Can you work these out from the model? Positions are in its coordinate system, mm. Face numbers are marked on the shaded views. Coordinates: 2 decimals unless noted, no trailing zeros. Order: outer loops, then holes, each group sorted by start corner. A loop starts at its lowest first (then second) coordinate and runs counter-clockwise, first axis right, second up. Notation, with made-up numbers: (74.25, 72) - (111.25, 72) arc R15 ccw to (111.25, 93) - close; hole circle Ø8 at (-5.5, 28.25). An arc over 180 degrees is marked (long way). Return JSON: item names as keys, results as strings. Group by question number.
1) Imagine slicing it at C-C (y = -5). Write out the boundary of the cut face in (x, z).
2) Imagine slicing it at B-B (x = 2.5). Write out the boundary of the cut face in (y, z), and give its area (3 significant figures).
3) Imagine slicing it at A-A (z = 5). Write out the boundary of the cut face in (x, y), and give its area (3 significant figures).
4) Imagine slicing it at D-D (z = 7.5). Write out the boundary of the cut face in (x, y), and give its area (3 significant figures).
5) If we mould it in two halves opening along X, with no side actions, what happens to the marked faces 1, 2 and 3? For each: pulls with the +X half, pulls with the -X half, needs draft (parallel to the pull), parting line crosses it, or undercut.
6) If I drill on line 1 along Y through (x, z) = (7.5, 5.5); line 2 along X through (y, z) = (-5, 3.25); line 3 along X through (y, z) = (-5, 4.75), over which ranges is the centre line in solid material (lowest first)?
```python
from build123d import *

# Parameters (mm, degrees)
ESQUISSE1_W             = 12
ESQUISSE1_H             = 10
BOSS_EXTRU_1_DEPTH      = 10
ESQUISSE2_R             = 3
ENL_V_MAT_EXTRU_2_DEPTH = 11
ESQUISSE3_R             = 1
ENL_V_MAT_EXTRU_3_DEPTH = 11


with BuildPart() as part:
    # Esquisse1 → Boss.-Extru.1 (new body)
    with BuildSketch(Plane.XY):
        with Locations((6, -5)):
            Rectangle(ESQUISSE1_W, ESQUISSE1_H)
    extrude(amount=BOSS_EXTRU_1_DEPTH)

    # Esquisse2 → Enlèv. mat.-Extru.2 (cut, through all)
    with BuildSketch(Plane.XY):
        with Locations((7.5, -5)):
            Circle(ESQUISSE2_R)
    extrude(amount=ENL_V_MAT_EXTRU_2_DEPTH, mode=Mode.SUBTRACT)

    # Esquisse3 → Enlèv. mat.-Extru.3 (cut, through all)
    with BuildSketch(Plane(origin=(0, 0, 0), x_dir=(1, 0, 0), z_dir=(0, 1, 0))):
        with Locations((2.5, -5)):
            Circle(ESQUISSE3_R)
    extrude(amount=-ENL_V_MAT_EXTRU_3_DEPTH, mode=Mode.SUBTRACT)


solid = part.part
```
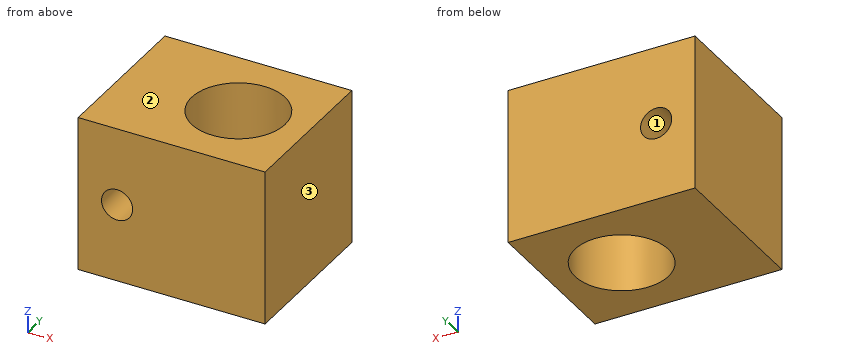
Calculated:
{
 "1": {"outline": "(0, 0) - (4.5, 0) - (4.5, 10) - (0, 10) - close; (10.5, 0) - (12, 0) - (12, 10) - (10.5, 10) - close; hole circle Ø2 at (2.5, 5)"},
 "2": {"outline": "(-10, 0) - (0, 0) - (0, 4) - (-10, 4) - close; (-10, 6) - (0, 6) - (0, 10) - (-10, 10) - close", "area": "80.0 mm2"},
 "3": {"outline": "(0, -10) - (1.5, -10) - (1.5, 0) - (0, 0) - close; (3.5, -10) - (12, -10) - (12, 0) - (3.5, 0) - close; hole circle Ø6 at (7.5, -5)", "area": "71.7 mm2"},
 "4": {"outline": "(0, -10) - (12, -10) - (12, 0) - (0, 0) - close; hole circle Ø6 at (7.5, -5)", "area": "91.7 mm2"},
 "5": {"face 1": "undercut", "face 2": "needs draft", "face 3": "pulls with the +X half"},
 "6": {"line 1": "-10 to -8, -2 to 0", "line 2": "0 to 4.5, 10.5 to 12", "line 3": "0 to 1.53, 3.47 to 4.5, 10.5 to 12"}
}
